```python
from build123d import *

# Parameters (mm, degrees)
F0_W     = 41
F0_H     = 51.442152
F1_DEPTH = 61
F2_W     = 34.694057
F2_H     = 36.070803
F3_DEPTH = 2
F4_W     = 8.398162
F4_H     = 8.535839
F5_DEPTH = 1.5


with BuildPart() as f1:
    # F0 (on Top) → F1 (new body)
    with BuildSketch(Plane.XY):
        with Locations((13.462494, -30.967161)):
            Rectangle(F0_W, F0_H)
    extrude(amount=F1_DEPTH)

    # F2 (on face) → F3 (join)
    with BuildSketch(Plane(origin=(0, -5.246085, 0), x_dir=(-1, 0, 0), z_dir=(0, 1, 0))):
        with Locations((-13.354457, 36.070805)):
            Rectangle(F2_W, F2_H)
    extrude(amount=F3_DEPTH)

    # F4 (on face) → F5 (join)
    with BuildSketch(Plane(origin=(0, -3.246085, 0), x_dir=(-1, 0, 0), z_dir=(0, 1, 0))):
        with Locations((-20.031688, 39.099652)):
            Rectangle(F4_W, F4_H)
        with Locations((-6.677231, 39.099652)):
            Rectangle(F4_W, F4_H)
    extrude(amount=F5_DEPTH)


solid = f1.part
```
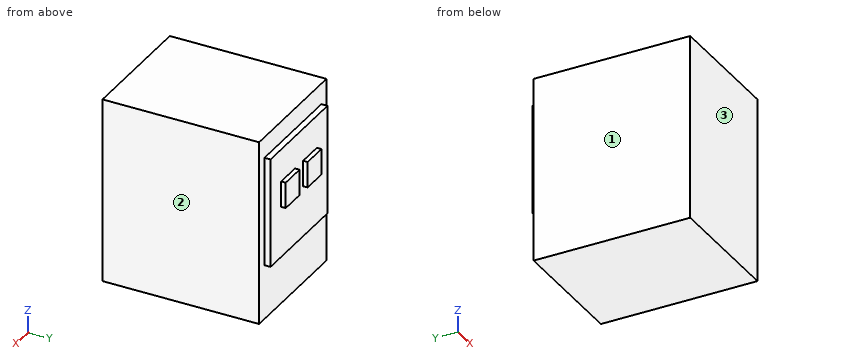
Can you work these out from the model? Positions are in its coordinate system, mm. Face numbers are marked on the shaded views. Round coordinates to 2 decimals unless told otherwise and drop trailing zeros. Loops run counter-clockwise (first coordinate to the right, second up) from the corner with the lowest first, then second, coordinate; pieces in that order, holes last.
Item 1: Suppose I cut it at D-D, the plane z = 36.5. Write out the boundary of the cut face in (x, y), then the cut area to 3 significant figures.
Item 2: Suppose I cut it at B-B, the plane z = 21. Write out the boundary of the cut face in (x, y).
Item 3: If we mould it in two halves opening along X, with no side actions, what happens to the marked faces 1, 2 and 3? For each: +X half, -X half, draft (parallel to the pull), parting line (faces both ways), or undercut.
Item 4: Suppose I cut it at A-A, the plane x = 13.5. Write out the boundary of the cut face in (y, z), then the cut area to 3 significant figures.
Item 5: Please list where these lines run through material, in increasing order: L1, parallel to Y at x = 6.5, z = 58; L2, parallel to Y at x = 12.5, z = 42.5.
Item 6: Will these pins go through, and if not, where does the flat tip stop? pin 1 Ø1.6 at (y, z) = (-2.5, 40) entering from +X; pin 2 Ø1.2 at (x, y) = (18.5, -2) entering from -Z; pin 3 Ø1 at (x, y) = (14, -4.5) entering from -Z; pin 4 Ø1 at (x, y) = (-0.5, -47.5) entering from -Z.
Item 7: Suppose I cut it at C-C, the plane x = 20. Write out the boundary of the cut face in (y, z).
Reported:
1. outline: (-7.04, -56.69) - (33.96, -56.69) - (33.96, -5.25) - (30.7, -5.25) - (30.7, -3.25) - (24.23, -3.25) - (24.23, -1.75) - (15.83, -1.75) - (15.83, -3.25) - (10.88, -3.25) - (10.88, -1.75) - (2.48, -1.75) - (2.48, -3.25) - (-3.99, -3.25) - (-3.99, -5.25) - (-7.04, -5.25) - close
1. area: 2,200 mm2
2. outline: (-7.04, -56.69) - (33.96, -56.69) - (33.96, -5.25) - (30.7, -5.25) - (30.7, -3.25) - (-3.99, -3.25) - (-3.99, -5.25) - (-7.04, -5.25) - close
3. face 1: -X half
3. face 2: +X half
3. face 3: draft
4. outline: (-56.69, 0) - (-5.25, 0) - (-5.25, 18.04) - (-3.25, 18.04) - (-3.25, 54.11) - (-5.25, 54.11) - (-5.25, 61) - (-56.69, 61) - close
4. area: 3,210 mm2
5. L1: y = -56.69 to -5.25
5. L2: y = -56.69 to -3.25
6. pin 1: stops at x = 30.7
6. pin 2: stops at z = 34.83
6. pin 3: stops at z = 18.04
6. pin 4: stops at z = 0
7. outline: (-56.69, 0) - (-5.25, 0) - (-5.25, 18.04) - (-3.25, 18.04) - (-3.25, 34.83) - (-1.75, 34.83) - (-1.75, 43.37) - (-3.25, 43.37) - (-3.25, 54.11) - (-5.25, 54.11) - (-5.25, 61) - (-56.69, 61) - close
